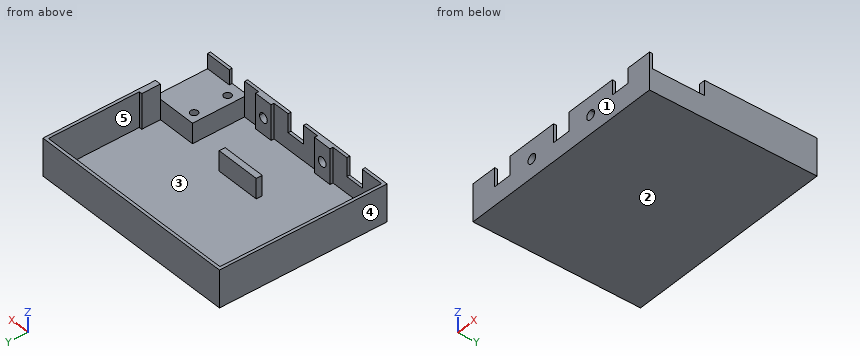
```python
from build123d import *

# Parameters (mm, degrees)
F0_W     = 12
F0_H     = 1.6
F0_H_2   = 7
F0_R     = 1
F1_DEPTH = 0.6
F2_W     = 12
F2_H     = 1.6
F2_H_2   = 7
F2_R     = 1
F3_DEPTH = 5.4
F4_W     = 2.5
F4_H     = 0.8
F4_W_2   = 0.8
F4_H_2   = 5
F5_DEPTH = 9.4
F6_DEPTH = 4.4
F7_DEPTH = 1
F8_R     = 1.25
F9_DEPTH = 1.6


# Not quite as in the source:
# - a feature names something its author has since deleted; it is built from what else it names


with BuildPart() as f1:
    # F0 (on Top) → F1 (new body)
    with BuildSketch(Plane.XY):
        Polygon((-57.15, 0), (-12, 0), (-12, 7), (-12, 14), (0, 14), (0, 43), (-22.575, 43), (-22.575, 41.4), (-34.575, 41.4), (-34.575, 43), (-57.15, 43), align=None)
        with Locations((-28.575, 15.6)):
            Rectangle(F0_W, F0_H, mode=Mode.SUBTRACT)
        Polygon((-57.15, 45), (-57.15, 43), (-34.575, 43), (-22.575, 43), (0, 43), (0, 45), align=None)
        with Locations((-6, 10.5)):
            Rectangle(F0_W, F0_H_2)
        with Locations((-9.5, 11.5)):
            Circle(F0_R, mode=Mode.SUBTRACT)
        with Locations((-6, 3.5)):
            Rectangle(F0_W, F0_H_2)
        with Locations((-9.5, 2.5)):
            Circle(F0_R, mode=Mode.SUBTRACT)
        with Locations((-28.575, 42.2)):
            Rectangle(F0_W, F0_H)
        with Locations((-28.575, 15.6)):
            Rectangle(F0_W, F0_H)
        with Locations((-9.5, 11.5)):
            Circle(F0_R)
        with Locations((-9.5, 2.5)):
            Circle(F0_R)
    extrude(amount=F1_DEPTH)

    # F2 (on face) → F3 (join)
    with BuildSketch(Plane.XY.offset(0.6)):
        with Locations((-28.575, 42.2)):
            Rectangle(F2_W, F2_H)
        with Locations((-28.575, 15.6)):
            Rectangle(F2_W, F2_H)
        with Locations((-6, 11.3)):
            Rectangle(F2_W, F2_H_2)
        with Locations((-9.5, 12.3)):
            Circle(F2_R, mode=Mode.SUBTRACT)
        with Locations((-6, 4.3)):
            Rectangle(F2_W, F2_H_2)
        with Locations((-9.5, 3.3)):
            Circle(F2_R, mode=Mode.SUBTRACT)
    extrude(amount=F3_DEPTH)

    # F4 (on face) → F5 (join)
    with BuildSketch(Plane.XY.offset(0.6)):
        Polygon((-45.125, 0.8), (-45.125, 0), (-31.075, 0), (-31.075, 0.8), (-35.6, 0.8), (-38.1, 0.8), (-40.6, 0.8), align=None)
        with Locations((-36.85, 1.2)):
            Rectangle(F4_W, F4_H)
        with Locations((-39.35, 1.2)):
            Rectangle(F4_W, F4_H)
        Polygon((-21.55, 1.6), (-21.55, 0.8), (-16.55, 0.8), (-16.55, 1.6), (-19.05, 1.6), align=None)
        Polygon((-26.075, 0.8), (-26.075, 0), (-12.025, 0), (-12.025, 0.8), (-16.55, 0.8), (-21.55, 0.8), align=None)
        Polygon((0, 0), (0, 0.8), (-0.8, 0.8), (-7.025, 0.8), (-7.025, 0), align=None)
        Polygon((0, 45), (-57.15, 45), (-57.15, 0), (-50.125, 0), (-50.125, 0.8), (-56.35, 0.8), (-56.35, 44.2), (-0.8, 44.2), (-0.8, 19.8), (-0.8, 14.8), (0, 14.8), align=None)
        with Locations((-1.2, 17.3)):
            Rectangle(F4_W_2, F4_H_2)
    extrude(amount=F5_DEPTH)

    # F4 (on face) → F6 (join)
    with BuildSketch(Plane.XY.offset(0.6)):
        Polygon((-31.075, 0.8), (-31.075, 0), (-26.075, 0), (-26.075, 0.8), (-28.575, 0.8), align=None)
        Polygon((-50.125, 0.8), (-50.125, 0), (-45.125, 0), (-45.125, 0.8), (-47.625, 0.8), align=None)
        Polygon((-12.025, 0), (-7.025, 0), (-7.025, 0.8), (-9.525, 0.8), (-12, 0.8), (-12.025, 0.8), align=None)
    extrude(amount=F6_DEPTH)

    # F7 (add): a face of the model
    f7_faces = [f1.faces().sort_by_distance(p)[0] for p in [
        (-9.525, 0.4, 5),
    ]]
    extrude(f7_faces, amount=F7_DEPTH)

    # F8 (on face) → F9 (cut)
    with BuildSketch(Plane.XZ):
        with Locations((-38.1, 5)):
            Circle(F8_R)
        with BuildLine():
            ThreePointArc((-17.8, 5), (-18.1661165235, 5.8838834765), (-19.05, 6.25))
            ThreePointArc((-19.05, 6.25), (-19.9338834765, 4.1161165235), (-17.8, 5))
        make_face()
    extrude(amount=-F9_DEPTH, mode=Mode.SUBTRACT)


solid = f1.part
```
Work out the finished part from the listing and answer in its coordinate system (mm). Face numbers are marked on the shaded views. A direction names the side the tool comes from. Round coordinates to 2 decimals unless told otherwise and drop trailing zeros. Order: outer loops, then holes, each group sorted by start corner. A loop starts at its lowest first (then second) coordinate and runs counter-clockwise, first axis right, second up.
Q1. A cutting plane is placed at D-D, the plane x = -9.5. Determine the outline of the cut face in (y, z).
Solution:
outline: (0, 0) - (45, 0) - (45, 10) - (44.2, 10) - (44.2, 0.6) - (14.8, 0.6) - (14.8, 6) - (13.3, 6) - (13.3, 0.6) - (11.3, 0.6) - (11.3, 6) - (4.3, 6) - (4.3, 0.6) - (2.3, 0.6) - (2.3, 6) - (0, 6) - close
Q2. Given pin 1 Ø1 at (x, y) = (-10, 3.5) entering from +Z, flat-ended and moving along its own axis, determine where the tip first touches the part or whether it passes through.
Solution:
pin 1: stops at z = 6
Q3. A cutting plane is placed at C-C, the plane y = 33.5. Determine the outline of the cut face in (x, z).
Solution:
outline: (-57.15, 0) - (0, 0) - (0, 10) - (-0.8, 10) - (-0.8, 0.6) - (-56.35, 0.6) - (-56.35, 10) - (-57.15, 10) - close
Q4. A cutting plane is placed at A-A, the plane z = 1.5. Count the separate pieces of the cut face and the enclosed holes in it, then the cut area to 3 significant figures.
Solution:
separate pieces: 3
enclosed holes: 3
area: 362 mm2
Q5. The mould has two halves that part along Y. Classify the marked faces 1, 2 and 3: pulls with the +Y half, pulls with the -Y half, needs draft (parallel to the pull), parting line crosses it, or undercut.
Solution:
face 1: pulls with the -Y half
face 2: needs draft
face 3: undercut
Q6. A tool of negligible diameter and unlimited length cuts with its end or side. For the marked faces 4 and 5, from which of +Z, -Z, +X, -X, +Y, -Y can it reach the whole face along a straight path? Write none if from no direction.
Solution:
face 4: +Z, -Z, -X, +Y, -Y
face 5: +Z
Q7. A cutting plane is placed at B-B, the plane x = -38.1. Determine the outline of the cut face in (y, z).
Solution:
outline: (0, 0) - (45, 0) - (45, 10) - (44.2, 10) - (44.2, 0.6) - (1.6, 0.6) - (1.6, 3.75) - (0, 3.75) - close; (0, 6.25) - (1.6, 6.25) - (1.6, 10) - (0, 10) - close
Q8. Find the intervals of material crossed by line 1 along Y through (x, z) = (-9.5, 1.75); line 2 along Z through (x, y) = (-38.1, 0.7); line 3 along X through (y, z) = (25, 9.25), in increasing order.
Solution:
line 1: y = 0 to 2.3, 4.3 to 11.3, 13.3 to 14.8, 44.2 to 45
line 2: z = 0 to 3.75, 6.25 to 10
line 3: x = -57.15 to -56.35, -0.8 to 0
